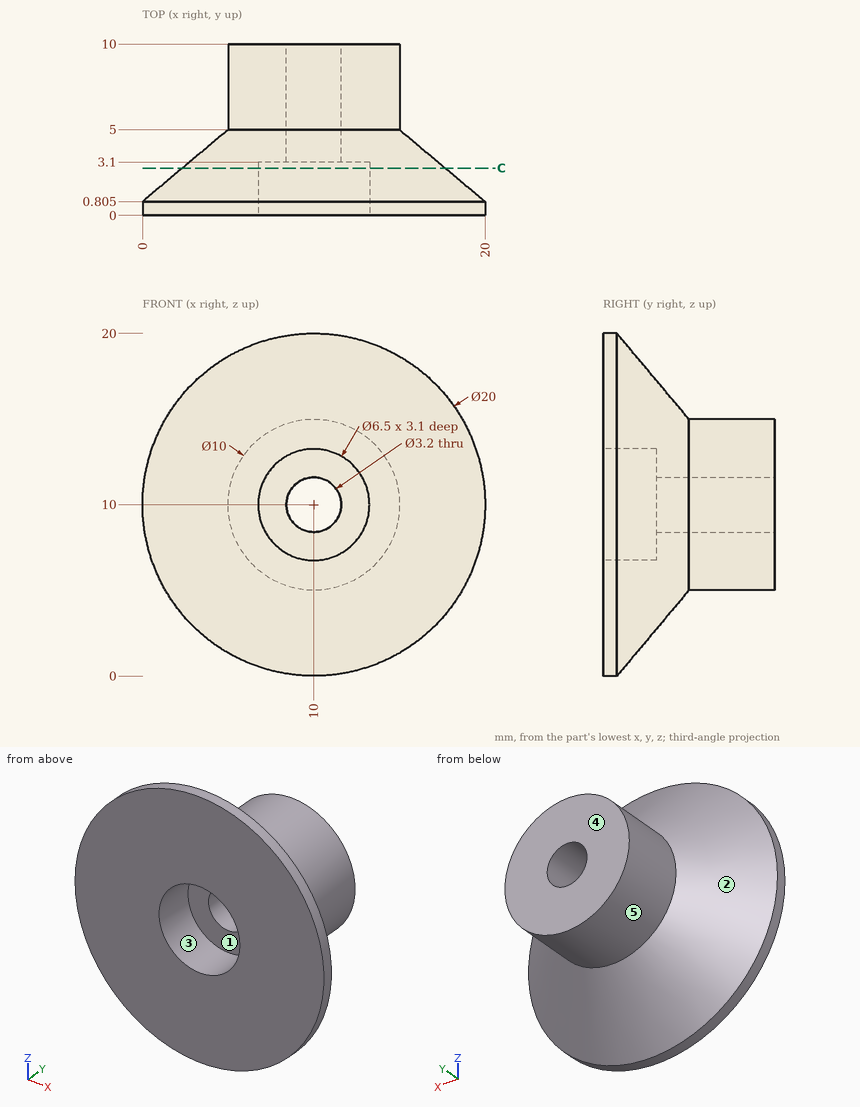
Job drawing, mm, ordinate dimensions from the low corner. One solid piece. A direction names the side the tool comes from. Give positions to 0.01 mm unless a question says otherwise; leave off trailing zeros. Write each loop counter-clockwise with the first axis right and the second up, starting at its lowest first coordinate (ties: lowest second). Pieces come first, ordered by that corner, then holes. Notation, with made-up numbers: (31, 64.25) - (67, 64.25) arc R15 cw to (67, 88.25) - close; hole circle Ø9 at (4, -6). An arc over 180 degrees is marked (long way). Answer as CSV lines item,"result".
1. 3-axis set-ups, long thin cutter, end or side, ignore diameter. For the marked faces 1 and 2: which of +Z, -Z, +X, -X, +Y, -Y reach the whole face in a straight line?
Responses:
face 1,"-Y"
face 2,"+Y"
2. Two-plate mould, pull along Z, no slides. Class the marked faces 3, 4 and 5: +Z half, -Z half, draft (parallel to the pull), parting line (faces both ways), or undercut.
Responses:
face 3,"undercut"
face 4,"draft"
face 5,"parting line"
3. Band-saw the part on C-C (y = 2.75). Write the cut outline in (x, z), and give its area (3 significant figures).
Responses:
outline,"circle Ø15.36 at (10, 10); hole circle Ø6.5 at (10, 10)"
area,"152 mm2"
4. Drill centre lines: L1, parallel to Z at x = 10, y = 6; L2, parallel to Z at x = 10.5, y = 5.75 (1 decimal); L3, parallel to X at y = 8.5, z = 8.75. Where is each one in solid material? Low to high. Write a range as [from, to].
Responses:
L1,"z = [5, 8.4], [11.6, 15]"
L2,"z = [5, 8.5], [11.5, 15]"
L3,"x = [5.16, 9], [11, 14.84]"
5. Pin check, flat tips, straight feed: pin 1 (7.5 mm diameter, centred on x = 10, z = 10, fed in from +Y); pin 2 (2 mm diameter, centred on x = 10, y = 7, fed in from -Z); pin 3 (6 mm diameter, centred on x = 15.5, y = 6.5, fed in from -Z); pin 4 (3.5 mm diameter, centred on x = 10, z = 10, fed in from -Y). Stop position of each tip, or through.
Responses:
pin 1,"stops at y = 10"
pin 2,"stops at z = 5"
pin 3,"stops at z = 5.12"
pin 4,"stops at y = 3.1"
